```python
from build123d import *

# Parameters (mm, degrees)
F0_R      = 60
F1_DEPTH  = 25
F2_R      = 45
F3_DEPTH  = 2
F4_R      = 11
F5_DEPTH  = 7
F6_R      = 45
F7_DEPTH  = 2
F8_R      = 11
F9_DEPTH  = 7
F10_R     = 8.5
F11_DEPTH = 25
F12_R     = 12.49999
F16_DEPTH = 25


# Not quite as in the source:
# - a fillet or chamfer is up to 0.001 mm smaller than in the source, because OpenCascade refuses the exact size


with BuildPart() as f1:
    # F0 (on Top) → F1 (new body)
    with BuildSketch(Plane.XY):
        Circle(F0_R)
    extrude(amount=F1_DEPTH)

    # F2 (on face) → F3 (cut)
    with BuildSketch(Plane.XY.offset(25)):
        Circle(F2_R)
    extrude(amount=-F3_DEPTH, mode=Mode.SUBTRACT)

    # F4 (on face) → F5 (cut)
    with BuildSketch(Plane.XY.offset(23)):
        Circle(F4_R)
    extrude(amount=-F5_DEPTH, mode=Mode.SUBTRACT)

    # F6 (on face) → F7 (cut)
    with BuildSketch(Plane(origin=(0, 0, 0), x_dir=(1, 0, 0), z_dir=(0, 0, -1))):
        Circle(F6_R)
    extrude(amount=-F7_DEPTH, mode=Mode.SUBTRACT)

    # F8 (on face) → F9 (cut)
    with BuildSketch(Plane(origin=(0, 0, 2), x_dir=(1, 0, 0), z_dir=(0, 0, -1))):
        Circle(F8_R)
    extrude(amount=-F9_DEPTH, mode=Mode.SUBTRACT)

    # F10 (on face) → F11 (cut)
    with BuildSketch(Plane(origin=(0, 0, 9), x_dir=(1, 0, 0), z_dir=(0, 0, -1))):
        Circle(F10_R)
    extrude(amount=-F11_DEPTH, mode=Mode.SUBTRACT)

    # F12 (radius 12.5 in the source; OpenCascade refuses exactly that, so slightly less here)
    f12_edges = [f1.edges().sort_by_distance(p)[0] for p in [
        (-60, 0, 25),
        (-60, 0, 0),
    ]]
    fillet(f12_edges, radius=F12_R)

    # F15 (on face) → F16 (cut)
    with BuildSketch(Plane.XY.offset(23)):
        with BuildLine():
            Line((-23.7309150398, -31.4583554864), (-11.8406927213, -9.2094279826))
            ThreePointArc((-11.8406927213, -9.2094279826), (-24.1709240611, -0.1529805421), (-39.4689776003, 0))
            ThreePointArc((-39.4689776003, 0), (-35.1668885168, -17.5136562569), (-23.7309150398, -31.4583554864))
        make_face()
        with BuildLine():
            Line((11.6958646104, -37.6011095941), (0, -15.4828215018))
            ThreePointArc((0, -15.4828215018), (-12.8825559704, -21.5513966495), (-18.4614025056, -34.6534699202))
            ThreePointArc((-18.4614025056, -34.6534699202), (-3.6886632813, -39.2568911162), (11.6958646104, -37.6011095941))
        make_face()
        with BuildLine():
            Line((38.0679219961, -10.3157823905), (16.2651948631, -10.3157823905))
            ThreePointArc((16.2651948631, -10.3157823905), (12.2364949642, -22.929504934), (18.3915793896, -34.6534699202))
            ThreePointArc((18.3915793896, -34.6534699202), (30.8515845586, -24.6043058224), (38.0679219961, -10.3157823905))
        make_face()
        with BuildLine():
            Line((29.1008390486, 26.5384856611), (15.2093013749, 6.5587405115))
            ThreePointArc((15.2093013749, 6.5587405115), (24.360120091, -4.7843640185), (38.8653166592, -6.1995587312))
            ThreePointArc((38.8653166592, -6.1995587312), (37.7282086233, 11.2864894274), (29.1008390486, 26.5384856611))
        make_face()
        with BuildLine():
            Line((-12.5216757879, 37.253908813), (0, 16.3887739182))
            ThreePointArc((0, 16.3887739182), (14.7450774696, 19.4214078257), (22.6965453476, 32.2037525475))
            ThreePointArc((22.6965453476, 32.2037525475), (5.7090018341, 39.0634462479), (-12.5216757879, 37.253908813))
        make_face()
        with BuildLine():
            Line((-38.4788028896, 8.5062459111), (-11.8609527126, 10.3406049311))
            ThreePointArc((-11.8609527126, 10.3406049311), (-11.4093820553, 23.6626254803), (-19.6125917137, 34.1691710055))
            ThreePointArc((-19.6125917137, 34.1691710055), (-31.7739639836, 23.3434055945), (-38.4788028896, 8.5062459111))
        make_face()
    extrude(amount=-F16_DEPTH, mode=Mode.SUBTRACT)


solid = f1.part
```
Geometry: final body of the model. Coordinates: model frame, mm. A direction names the side the tool comes from. Round coordinates to 2 decimals unless told otherwise and drop trailing zeros. Order: outer loops, then holes, each group sorted by start corner. A loop starts at its lowest first (then second) coordinate and runs counter-clockwise, first axis right, second up. Notation, with made-up numbers: M 27,-32.5 L 65,-32.5 A15 cw 65,-26.5 Z; hole C 47,34 d2. An arc over 180 degrees is marked long. Use one line per item in the form item = value. Start each with the question number.
Q1. Material intervals for line 1 (Y direction, x = 6, z = 4.25); line 2 (X direction, y = 25, z = 10.25); line 3 (Y direction, x = -15.5, z = 20.25), sorted ascending. Write a range as [from, to].
Q2. Pin query (flat end, axial travel): pin 1 Ø1.5 at (x, z) = (24.5, 18) entering from +Y; pin 2 Ø1.5 at (y, z) = (39, 6.5) entering from +X; pin 3 Ø5 at (x, z) = (28.5, 3) entering from -Y. Return the tip coordinate at first contact, or that it passes through.
Q3. Cut plane B-B (x = -16). Count the separate pieces of the cut face and the enclosed holes in it, and give its area (3 significant figures).
Q4. Cut plane A-A (z = 20.25). Return loops of the section in (x, y).
Q5. Access query for faces 1 (the face through (20.765, 39.923, 0.986)), 2 (the face through (-17.87, -20.49, 12.65)), 3 (the face through (9, -9, 23)). Directions: +Z, -Z, +X, -X, +Y, -Y. A direction counts if a zero-diameter tool reaches every point of the face in a straight line with its end or side. Return the directions, or none.
Geometry results:
q1.line_1 = [-56.57, -38.96], [-26.83, -9.22], [9.22, 16.12], [39.02, 56.57]
q1.line_2 = [-54.32, -30.49], [-11.9, -5.17], [20.04, 28.03], [30.43, 54.32]
q1.line_3 = [-55.17, -36.13], [-24.93, -16.06], [-5.16, 10.09], [30.72, 55.17]
q2.pin_1 = 53.88
q2.pin_2 = 44.4
q2.pin_3 = -50.77
q3.separate_pieces = 4
q3.enclosed_holes = 0
q3.area = 1,500 mm^2
q4.outline = C 0,0 d114.62; hole M -39.47,0 A40.77 ccw -23.73,-31.46 L -11.84,-9.21 A24.94 ccw Z; hole M -38.48,8.51 L -11.86,10.34 A19.52 ccw -19.61,34.17 A39.14 ccw Z; hole M -18.46,-34.65 A38.07 ccw 11.7,-37.6 L 0,-15.48 A20 ccw Z; hole M -12.52,37.25 L 0,16.39 A19.07 ccw 22.7,32.2 A38.32 ccw Z; hole C 0,0 d22; hole M 15.21,6.56 A18.83 ccw 38.87,-6.2 A39.28 ccw 29.1,26.54 Z; hole M 16.27,-10.32 A17.15 ccw 18.39,-34.65 A38 ccw 38.07,-10.32 Z
q5.face_1 = -Z
q5.face_2 = +Z, -Z
q5.face_3 = +Z
